```python
from build123d import *

# Parameters (mm, degrees)
F0_W     = 152.4
F0_H     = 12.7
F1_DEPTH = 165.1
F2_SIZE2 = 76.2
F2_SIZE  = 101.6
F3_W     = 78.9234735198
F3_H     = 88.9
F4_DEPTH = 19.812
F6_DEPTH = 25.4


with BuildPart() as f1:
    # F0 (on Top) → F1 (new body)
    with BuildSketch(Plane.XY):
        Rectangle(F0_W, F0_H)
    extrude(amount=F1_DEPTH)

    # F2
    f2_edges = [f1.edges().sort_by_distance(p)[0] for p in [
        (76.2, 0, 0),
    ]]
    f2_side = f1.faces().sort_by_distance((0, 0, 0))[0]
    chamfer(f2_edges, length=F2_SIZE, length2=F2_SIZE2, reference=f2_side)

    # F3 (on face) → F4 (join)
    with BuildSketch(Plane.XZ.offset(6.35)):
        with Locations((36.7382632401, 120.65)):
            Rectangle(F3_W, F3_H)
    extrude(amount=F4_DEPTH)

    # F5 (on face) → F6 (cut)
    with BuildSketch(Plane(origin=(0, 6.35, 0), x_dir=(-1, 0, 0), z_dir=(0, 1, 0))):
        Polygon((-8.4666666667, 76.2), (-76.2, 76.2), (-8.4666666667, 25.4), align=None)
    extrude(amount=-F6_DEPTH, mode=Mode.SUBTRACT)


solid = f1.part
```
Design review of the part built by this model. Coordinates are the model's own, in mm. A direction names the side the tool comes from. Give positions to 0.01 mm unless a question says otherwise; leave off trailing zeros. Write each loop counter-clockwise with the first axis right and the second up, starting at its lowest first coordinate (ties: lowest second). Pieces come first, ordered by that corner, then holes. Notation, with made-up numbers: (-24.5, -11.5) - (23.5, -11.5) arc R14 ccw to (23.5, -5.5) - close; hole circle Ø9 at (82.25, -26). An arc over 180 degrees is marked (long way). Return JSON: item names as keys, results as strings. Group by question number.
(1) We need section B-B, the plane y = 3. Give the boundary of the cut face in (x, z), then the cut area to 3 significant figures.
(2) To check wall thickness, follow probe 1 along X at (y, z) = (-23, 111); probe 2 along Y at (x, z) = (-35, 158); probe 3 along Z at (x, y) = (13.5, -1). State the ranges of each line that lie inside material, in increasing order.
(3) We need section C-C, the plane x = 6. Give the boundary of the cut face in (y, z), then the cut area to 3 significant figures.
(4) Mouldability with a two-part tool opening along Z and no side actions: class faces 1 (the flat face through (-8.2, -0.1, 12.9)), 2 (the flat face through (16, -6, 165.1)), 3 (the flat face through (-76.2, 0, 81)) as +Z half, -Z half, draft (parallel to the pull), parting line (faces both ways), or undercut.
(5) Insertion check: pin 1 (6.5 mm diameter, centred on y = -1.5, z = 48, fed in from +X); pin 2 (10 mm diameter, centred on x = 39.5, y = -9.5, fed in from -Z); pin 3 (6 mm diameter, centred on y = -19.5, z = 99.5, fed in from -X). Each pin has a flat end and moves straight along its axis. Give the tip position at first contact, or say it passes through.
(6) We need section D-D, the plane x = -54. Give the boundary of the cut face in (y, z).
(7) Machinability: for faces 4 (the flat face through (-2.723, -16, 120)), 5 (the flat face through (8.467, 0, 50)), 6 (the flat face through (-18, 6.35, 100)), which of the approach directions +Z, -Z, +X, -X, +Y, -Y give a long, thin tool a straight path to every point of the face, cutting with its end or side? Answer none if there is none.
(8) We need section A-A, the plane z = 81. Give the boundary of the cut face in (x, y).
Reported:
{
 "1": {"outline": "(-76.2, 0) - (-25.4, 0) - (8.47, 25.4) - (8.47, 76.2) - (76.2, 76.2) - (76.2, 165.1) - (-76.2, 165.1) - close", "area": "19,600 mm2"},
 "2": {"probe 1": "x = -2.72 to 76.2", "probe 2": "y = -6.35 to 6.35", "probe 3": "z = 76.2 to 165.1"},
 "3": {"outline": "(-26.16, 76.2) - (-6.35, 76.2) - (-6.35, 23.55) - (6.35, 23.55) - (6.35, 165.1) - (-26.16, 165.1) - close", "area": "3,560 mm2"},
 "4": {"face 1": "-Z half", "face 2": "+Z half", "face 3": "draft"},
 "5": {"pin 1": "stops at x = 8.47", "pin 2": "stops at z = 76.2", "pin 3": "stops at x = -2.72"},
 "6": {"outline": "(-6.35, 0) - (6.35, 0) - (6.35, 165.1) - (-6.35, 165.1) - close"},
 "7": {"face 4": "+Z, -Z, -X, -Y", "face 5": "-Z, +X, +Y, -Y", "face 6": "+Z, -Z, +X, -X, +Y"},
 "8": {"outline": "(-76.2, -6.35) - (-2.72, -6.35) - (-2.72, -26.16) - (76.2, -26.16) - (76.2, 6.35) - (-76.2, 6.35) - close"}
}
